The listing builds one solid part. Answer for the finished solid, in the listing's coordinates (mm). A direction names the side the tool comes from. Round coordinates to 2 decimals unless told otherwise and drop trailing zeros. Loops run counter-clockwise (first coordinate to the right, second up) from the corner with the lowest first, then second, coordinate; pieces in that order, holes last. Notation, with made-up numbers: M 20.25,-25 L 66.25,-25 A9 cw 66.25,-10 Z; hole C 8,-18 d4. An arc over 180 degrees is marked long. Put each result on its own line as item: value. Start each with the question number.
(1) Section A-A, the plane z = 11.5 is taken. Determine the outline of the cut face in (x, y).
(2) Which of the six approach directions +Z, -Z, +X, -X, +Y, -Y give full straight-line access (tool end or side, diameter ignored) to faces 1 (the face through (-22, 8, 23)), 2 (the face through (10, 10, 12)), 3 (the face through (-47, 10, 0)), 4 (the face through (-21, 10, -20.5))?
(3) Straight lines are drawn through the part: line 1 (Z direction, x = -15.5, y = 7); line 2 (X direction, y = 18.5, z = -9.5); line 3 (Y direction, x = -20.5, z = 21.8). For each, find the intervals that lie inside material, in ascending order.
(4) Determine the mould class of faces 5 (the face through (-23.82, 13.04, 28.04)), 6 (the face through (-49, 10, -4)), 7 (the face through (10, 10, -12)) for opening direction X: released by +X, released by -X, zero draft, split by the parting line, or undercut.
(5) Section D-D, the plane x = -20.5 is taken. Determine the outline of the cut face in (y, z).
(6) Flat-ended cylindrical pins translate along their axes: P1, Ø2.5, axis at y = 10.5, z = 0.5, coming from the +X side; P2, Ø6, axis at y = 11, z = 14, coming from the +X side; P3, Ø8, axis at x = 20.5, z = -15.5, coming from the -Y side; P4, Ø6, axis at y = 11, z = 0.5, coming from the -X side. Find the tip coordinate at first contact, or state that the pin passes through.
(7) Section B-B, the plane x = 18.5 is taken. Determine the outline of the cut face in (y, z).
(8) Section C-C, the plane y = 17 is taken. Determine the outline of the cut face in (x, z), then the cut area to 3 significant figures.
```python
from build123d import *

# Parameters (mm, degrees)
SKETCH1_W           = 41
SKETCH1_H           = 41
BOSS_EXTRUDE1_DEPTH = 20
SKETCH2_R           = 2.5
CUT_EXTRUDE1_DEPTH  = 40
SKETCH3_R           = 4.5
CUT_EXTRUDE2_DEPTH  = 5


with BuildPart() as part:
    # Sketch1 → Boss-Extrude1 (new body)
    with BuildSketch(Plane(origin=(0, 0, 0), x_dir=(1, 0, 0), z_dir=(0, 1, 0))):
        Polygon((-51, 30.5), (10, 30.5), (30, 30.5), (30, 20.5), (10, 20.5), (10, 4), (6, 4), (6, -4), (10, -4), (10, -20.5), (30, -20.5), (30, -30.5), (10, -30.5), (-51, -30.5), (-51, -4), (-47, -4), (-47, 4), (-51, 4), align=None)
        with Locations((-20.5, 0)):
            Rectangle(SKETCH1_W, SKETCH1_H, mode=Mode.SUBTRACT)
    extrude(amount=BOSS_EXTRUDE1_DEPTH)

    # Sketch2 → Cut-Extrude1 (cut)
    with BuildSketch(Plane.XY.offset(30.5)):
        with Locations((-20.5, 10)):
            Circle(SKETCH2_R)
    extrude(amount=-CUT_EXTRUDE1_DEPTH, mode=Mode.SUBTRACT)

    # Sketch3 → Cut-Extrude2 (cut)
    with BuildSketch(Plane.XY.offset(30.5)):
        with Locations((-20.5, 10)):
            Circle(SKETCH3_R)
    extrude(amount=-CUT_EXTRUDE2_DEPTH, mode=Mode.SUBTRACT)


solid = part.part
```
Recorded:
1. outline: M -51,0 L -41,0 L -41,20 L -51,20 Z; M 0,0 L 10,0 L 10,20 L 0,20 Z
2. face 1: +Z
2. face 2: +X, +Y, -Y
2. face 3: -X, +Y, -Y
2. face 4: +Y, -Y
3. line 1: z = -30.5 to -20.5, 20.5 to 30.5
3. line 2: x = -51 to -41, 0 to 10
3. line 3: y = 0 to 7.5, 12.5 to 20
4. face 5: undercut
4. face 6: zero draft
4. face 7: released by +X
5. outline: M 0,-30.5 L 20,-30.5 L 20,-20.5 L 0,-20.5 Z; M 0,20.5 L 7.5,20.5 L 7.5,25.5 L 5.5,25.5 L 5.5,30.5 L 0,30.5 Z; M 12.5,20.5 L 20,20.5 L 20,30.5 L 14.5,30.5 L 14.5,25.5 L 12.5,25.5 Z
6. P1: stops at x = 6
6. P2: stops at x = 10
6. P3: passes through
6. P4: stops at x = -47
7. outline: M 0,-30.5 L 20,-30.5 L 20,-20.5 L 0,-20.5 Z; M 0,20.5 L 20,20.5 L 20,30.5 L 0,30.5 Z
8. outline: M -51,-30.5 L 30,-30.5 L 30,-20.5 L 10,-20.5 L 10,-4 L 6,-4 L 6,4 L 10,4 L 10,20.5 L 30,20.5 L 30,30.5 L -51,30.5 L -51,4 L -47,4 L -47,-4 L -51,-4 Z; hole M -41,-20.5 L 0,-20.5 L 0,20.5 L -41,20.5 Z
8. area: 2,380 mm²
